from build123d import *

# Parameters (mm, degrees)
SKETCH_1_R      = 5.4
EXTRUDE_1_DEPTH = 4


with BuildPart() as part:
    # Эскиз1 → Бобышка-Вытянуть1 (new body)
    with BuildSketch(Plane.XY):
        with BuildLine():
            Line((-25, 24), (25, 24))
            Line((25, 24), (25, 21))
            Line((25, 21), (13.846153846, -5.769230769))
            ThreePointArc((13.846153846, -5.769230769), (0, -15), (-13.846153846, -5.769230769))
            Line((-13.846153846, -5.769230769), (-25, 21))
            Line((-25, 21), (-25, 24))
        make_face()
        Circle(SKETCH_1_R, mode=Mode.SUBTRACT)
    extrude(amount=EXTRUDE_1_DEPTH)


solid = part.part
Check sheet for the modelled part. Datum: model origin and axes. Units: mm. Round coordinates to 2 decimals unless told otherwise and drop trailing zeros. Order: outer loops, then holes, each group sorted by start corner. A loop starts at its lowest first (then second) coordinate and runs counter-clockwise, first axis right, second up.
(1) Go/stop test with flat-tipped pins: P1, Ø2, axis at x = 2, z = 3, coming from the -Y side; P2, Ø1, axis at y = 16.5, z = 2, coming from the -X side; P3, Ø2, axis at y = 16, z = 2, coming from the +X side. Record where each tip stops, or that it passes through.
(2) Cross-section at C-C, the plane x = -1.5. Enter the section's corners in (y, z).
(3) Cross-section at A-A, the plane z = 3.3. Enter the section's corners in (x, y).
(4) Cross-section at B-B, the plane y = 0. Enter the section's corners in (x, z).
(5) Scan lines: probe 1 along Y at (x, z) = (0, 2.55); probe 2 along Y at (x, z) = (-4, 1.5); probe 3 along X at (y, z) = (1, 1.4). Record each from-to range of solid material in increasing order.
(6) Cross-section at D-D, the plane y = -12. Enter the section's corners in (x, z), and give its area (3 significant figures).
(7) Draft check along Y on faces 1 (the cylindrical face through (0, -15, 2)), 2 (the cylindrical face through (-1.17, -5.27, 1.97)), 3 (the flat face through (25, 23, 2)), 4 (the flat face through (0, 24, 2)). Enter one of: pulls with the +Y half, pulls with the -Y half, needs draft (parallel to the pull), parting line crosses it, or undercut.
Check sheet entries:
1. P1: stops at y = -14.97
1. P2: stops at x = -23.33
1. P3: stops at x = 23.33
2. outline: (-14.92, 0) - (-5.19, 0) - (-5.19, 4) - (-14.92, 4) - close; (5.19, 0) - (24, 0) - (24, 4) - (5.19, 4) - close
3. outline: (-25, 21) - (-13.85, -5.77) arc R15 ccw to (13.85, -5.77) - (25, 21) - (25, 24) - (-25, 24) - close; hole circle Ø10.8 at (0, 0)
4. outline: (-16.25, 0) - (-5.4, 0) - (-5.4, 4) - (-16.25, 4) - close; (5.4, 0) - (16.25, 0) - (16.25, 4) - (5.4, 4) - close
5. probe 1: y = -15 to -5.4, 5.4 to 24
5. probe 2: y = -14.46 to -3.63, 3.63 to 24
5. probe 3: x = -16.67 to -5.31, 5.31 to 16.67
6. outline: (-9, 0) - (9, 0) - (9, 4) - (-9, 4) - close
6. area: 72.0 mm2
7. face 1: pulls with the -Y half
7. face 2: undercut
7. face 3: needs draft
7. face 4: pulls with the +Y half
